from build123d import *

# Parameters (mm, degrees)
SKETCH1_W           = 50
SKETCH1_H           = 53
BOSS_EXTRUDE1_DEPTH = 2
SKETCH2_W           = 50
SKETCH2_H           = 2
BOSS_EXTRUDE2_DEPTH = 62
SKETCH3_R           = 9.1
SKETCH3_R_2         = 2.6
SKETCH3_R_3         = 2.1
CUT_EXTRUDE1_DEPTH  = 2
CUT_EXTRUDE2_DEPTH  = 2
FILLET1_R           = 5


with BuildPart() as part:
    # Sketch1 → Boss-Extrude1 (new body)
    with BuildSketch(Plane(origin=(0, 0, 0), x_dir=(0, 1, 0), z_dir=(0, 0, 1))):
        Rectangle(SKETCH1_W, SKETCH1_H)
    extrude(amount=BOSS_EXTRUDE1_DEPTH)

    # Sketch2 → Boss-Extrude2 (add)
    with BuildSketch(Plane(origin=(0, 0, 0), x_dir=(0, 1, 0), z_dir=(0, 0, 1))):
        with Locations((0, -27.5)):
            Rectangle(SKETCH2_W, SKETCH2_H)
    extrude(amount=BOSS_EXTRUDE2_DEPTH)

    # Sketch3 → Cut-Extrude1 (cut)
    with BuildSketch(Plane(origin=(26.5, 0, 0), x_dir=(0, -1, 0), z_dir=(-1, 0, 0))):
        with Locations((0, 37)):
            Circle(SKETCH3_R)
        with Locations((16, 37)):
            Circle(SKETCH3_R_2)
        with Locations((-16, 37)):
            Circle(SKETCH3_R_2)
        with Locations((0, 51.5)):
            Circle(SKETCH3_R_3)
        with Locations((0, 22.5)):
            Circle(SKETCH3_R_3)
    extrude(amount=-CUT_EXTRUDE1_DEPTH, mode=Mode.SUBTRACT)

    # Sketch4 → Cut-Extrude2 (cut)
    with BuildSketch(Plane.XY.offset(2)):
        with BuildLine():
            Line((-11.5, 18.5), (-11.5, 7.5))
            ThreePointArc((-11.5, 7.5), (-14, 5), (-16.5, 7.5))
            Line((-16.5, 7.5), (-16.5, 18.5))
            ThreePointArc((-16.5, 18.5), (-14, 21), (-11.5, 18.5))
        make_face()
        with BuildLine():
            Line((-11.5, -7.5), (-11.5, -18.5))
            ThreePointArc((-11.5, -18.5), (-14, -21), (-16.5, -18.5))
            Line((-16.5, -18.5), (-16.5, -7.5))
            ThreePointArc((-16.5, -7.5), (-14, -5), (-11.5, -7.5))
        make_face()
        with BuildLine():
            Line((16.5, 18.5), (16.5, 7.5))
            ThreePointArc((16.5, 7.5), (14, 5), (11.5, 7.5))
            Line((11.5, 7.5), (11.5, 18.5))
            ThreePointArc((11.5, 18.5), (14, 21), (16.5, 18.5))
        make_face()
        with BuildLine():
            Line((16.5, -7.5), (16.5, -18.5))
            ThreePointArc((16.5, -18.5), (14, -21), (11.5, -18.5))
            Line((11.5, -18.5), (11.5, -7.5))
            ThreePointArc((11.5, -7.5), (14, -5), (16.5, -7.5))
        make_face()
    extrude(amount=-CUT_EXTRUDE2_DEPTH, mode=Mode.SUBTRACT)

    # Fillet1
    fillet1_edges = [part.edges().sort_by_distance(p)[0] for p in [
        (28.5, 0, 0),
        (27.5, -25, 62),
        (26.5, 0, 2),
        (27.5, 25, 62),
        (-26.5, -25, 1),
        (-26.5, 25, 1),
    ]]
    fillet(fillet1_edges, radius=FILLET1_R)


solid = part.part
Verification items for the finished model (mm, model axes). A direction names the side the tool comes from. Coordinates: 2 decimals unless noted, no trailing zeros. Write each loop counter-clockwise with the first axis right and the second up, starting at its lowest first coordinate (ties: lowest second). Pieces come first, ordered by that corner, then holes. Notation, with made-up numbers: M 84.25,33.5 L 112.25,33.5 A20 cw 112.25,59.5 Z; hole C 9.25,77.25 d8. An arc over 180 degrees is marked long. Use a Markdown table: item, result.
Q1. Go/stop test with flat-tipped pins: P1, Ø4, axis at y = 0, z = 51.5, coming from the +X side; P2, Ø2, axis at y = -14, z = 33, coming from the -X side; P3, Ø2, axis at y = 12, z = 1, coming from the +X side; P4, Ø4, axis at x = -8, y = -5.5, coming from the +Z side. Record where each tip stops, or that it passes through.
Reply:
| item | result |
|---|---|
| P1 | passes through |
| P2 | stops at x = 26.5 |
| P3 | stops at x = 27.5 |
| P4 | stops at z = 2 |
Q2. Set-up check for faces 5 (the face through (26.5, -6, 28)), 6 (the face through (-14, 21, 1)), 7 (the face through (27.5, -18.4, 36)): record each of +Z, -Z, +X, -X, +Y, -Y from which the full face is reachable in a straight line by a thin tool's end or side.
Reply:
| item | result |
|---|---|
| face 5 | +Z, -X, +Y, -Y |
| face 6 | +Z, -Z |
| face 7 | +X, -X |
Q3. Sectioned sample at A-A, the plane z = 22.5. Record the boundary of the cut face in (x, y).
Reply:
| item | result |
|---|---|
| outline | M 26.5,-25 L 28.5,-25 L 28.5,-2.1 L 26.5,-2.1 Z; M 26.5,2.1 L 28.5,2.1 L 28.5,25 L 26.5,25 Z |
Q4. Sectioned sample at C-C, the plane x = 14. Record the boundary of the cut face in (y, z), plus the area to 3 significant figures.
Reply:
| item | result |
|---|---|
| outline | M -25,0 L -21,0 L -21,2 L -25,2 Z; M -5,0 L 5,0 L 5,2 L -5,2 Z; M 21,0 L 25,0 L 25,2 L 21,2 Z |
| area | 36.0 mm² |
Q5. Draft check along Y on faces 1 (the face through (27, -24, 60)), 2 (the face through (-2, 0, 0)), 3 (the face through (27.49, -1.13, 24.27)), 4 (the face through (27, 23, 61)). Enter one of: +Y half, -Y half, draft (parallel to the pull), parting line (faces both ways), or undercut.
Reply:
| item | result |
|---|---|
| face 1 | -Y half |
| face 2 | draft |
| face 3 | undercut |
| face 4 | +Y half |
Q6. Sectioned sample at B-B, the plane y = 17. Record the boundary of the cut face in (x, z), plus the area to 3 significant figures.
Reply:
| item | result |
|---|---|
| outline | M -26.5,0 L -16.5,0 L -16.5,2 L -26.5,2 Z; M -11.5,0 L 11.5,0 L 11.5,2 L -11.5,2 Z; M 16.5,0 L 23.5,0 A5 ccw 28.5,5 L 28.5,34.6 L 26.5,34.6 L 26.5,7 A5 cw 21.5,2 L 16.5,2 Z; M 26.5,39.4 L 28.5,39.4 L 28.5,62 L 26.5,62 Z |
| area | 200 mm² |
Q7. Sectioned sample at D-D, the plane y = 10.5. Record the boundary of the cut face in (x, z), plus the area to 3 significant figures.
Reply:
| item | result |
|---|---|
| outline | M -26.5,0 L -16.5,0 L -16.5,2 L -26.5,2 Z; M -11.5,0 L 11.5,0 L 11.5,2 L -11.5,2 Z; M 16.5,0 L 23.5,0 A5 ccw 28.5,5 L 28.5,62 L 26.5,62 L 26.5,7 A5 cw 21.5,2 L 16.5,2 Z |
| area | 210 mm² |
Q8. Thickness scan on line 1 (X direction, y = -22, z = 34); line 2 (Z direction, x = 27.7, y = 0); line 3 (Z direction, x = 27.35, y = 16). Record the ranges inside material, lowest first.
Reply:
| item | result |
|---|---|
| line 1 | x = 26.5 to 28.5 |
| line 2 | z = 2.29 to 20.4, 24.6 to 27.9, 46.1 to 49.4, 53.6 to 62 |
| line 3 | z = 1.81 to 34.4, 39.6 to 62 |
